Model file for the job. Use its own axes, mm. Face numbers are marked on the shaded views. Round coordinates to 2 decimals unless told otherwise and drop trailing zeros. Write each loop counter-clockwise with the first axis right and the second up, starting at its lowest first coordinate (ties: lowest second). Pieces come first, ordered by that corner, then holes.
Autodesk Fusion 360 part; units mm, degrees
sketch "Sketch1" plane through (0, 0, 0) normal (0, 1, 0) x (1, 0, 0)
  line L0 (0, 0) -> (33.75, 0)
  line L1 (33.75, 0) -> (33.75, -6)
  line L2 (33.75, -6) -> (0, -6)
  line L3 (0, -6) -> (0, 0)
  line L4 (3, -3.9) -> (3, -2.1)
  line L5 (30.75, -2.1) -> (30.75, -3.9)
  line L6 (30.75, -3.9) -> (13.625, -3.9)
  line L7 (12.375, -3.9) -> (3, -3.9)
  line L8 (3, -2.1) -> (12.375, -2.1)
  line L9 (13.625, -2.1) -> (30.75, -2.1)
  arc A0 (12.375, -2.1) -> (13.625, -2.1) centre (13, -2.1) ccw
  arc A1 (12.625, 0) -> (13.375, 0) centre (13, 0) ccw
  arc A2 (13.375, -6) -> (12.625, -6) centre (13, -6) ccw
  arc A3 (13.625, -3.9) -> (12.375, -3.9) centre (13, -3.9) ccw
  dimension "d1" = 33.75
  dimension "d2" = 6
  dimension "d8" = 2.1
  dimension "d9" = 3
  dimension "d10" = 2.1
  dimension "d11" = 3
  dimension "d12" = 27
  dimension "d20" = 10
  dimension "d22" = 10
  dimension "d25" = 0.75
  dimension "d26" = 0.75
  dimension "d27" = 0.625
  dimension "d33" = 1.25
extrude "Extrude1" add sketch "Sketch1" along normal blind 11 contours L0 L1 L2 L3 A1 A2
sketch "Sketch2" plane through (0, 0, 0) normal (0, 0, -1) x (-1, 0, 0)
  line L0 (-33.75, 0) -> (0, 0)
  line L1 (0, 0) -> (0, 11)
  line L2 (0, 11) -> (-33.75, 11)
  line L3 (-33.75, 11) -> (-33.75, 0)
  arc A0 (0, 11) -> (0, 0) centre (12.5393, 5.5) ccw
  line L4 (0, 11) -> (0, 0)
  line L5 (-16.875, 11) -> (-16.875, 0)
  line L6 (-33.75, 11) -> (-33.75, 0)
  arc A1 (-33.75, 0) -> (-33.75, 11) centre (-46.2893, 5.5) ccw
  line L7 (-33.75, 0) -> (-33.75, 11)
extrude "Extrude2" cut sketch "Sketch2" against normal through all contours L3 L6 A1 L7 | L1 A0 L4
fillet "Fillet1" radius 1 2 edges at (0, 11, 3) (0, 0, 3)
fillet "Fillet1" radius 1 2 edges at (33.75, 11, 3) (33.75, 0, 3)
sketch "Sketch3" plane through (0, 11, 0) normal (0, 1, 0) x (-1, 0, 0)
  line L0 (-32.3029, 6) -> (-32.3029, 0)
  line L1 (-32.3029, 0) -> (-1.4471, 0)
  line L2 (-1.4471, 0) -> (-1.4471, 6)
  line L3 (-1.4471, 6) -> (-32.3029, 6)
  line L4 (-30.75, 3.9) -> (-13.625, 3.9)
  line L5 (-3, 3.9) -> (-3, 2.1)
  line L6 (-3, 2.1) -> (-12.375, 2.1)
  arc A0 (-12.375, 2.1) -> (-13.625, 2.1) centre (-13, 2.1) ccw
  line L7 (-13.625, 2.1) -> (-30.75, 2.1)
  line L8 (-30.75, 2.1) -> (-30.75, 3.9)
  circle A1 centre (-13, 0) radius 0.375
  circle A2 centre (-13, 6) radius 0.375
  arc A3 (-13.625, 3.9) -> (-12.375, 3.9) centre (-13, 3.9) ccw
  line L9 (-12.375, 3.9) -> (-3, 3.9)
  dimension "d28" = 0.75
  dimension "d29" = 0.75
  dimension "d30" = 10
  dimension "d31" = 10
extrude "Extrude3" cut sketch "Sketch3" against normal through all contours L3 A2 | L1 A1 picked at (-13.0916, 5.915) picked at (-12.9084, 0.085)
equation "d8 = d10"
equation "d11 = d9"
equation "d25 = d24"
equation "d26 = d24"
equation "d27 = d33 / 2"
equation "d31 = d30"
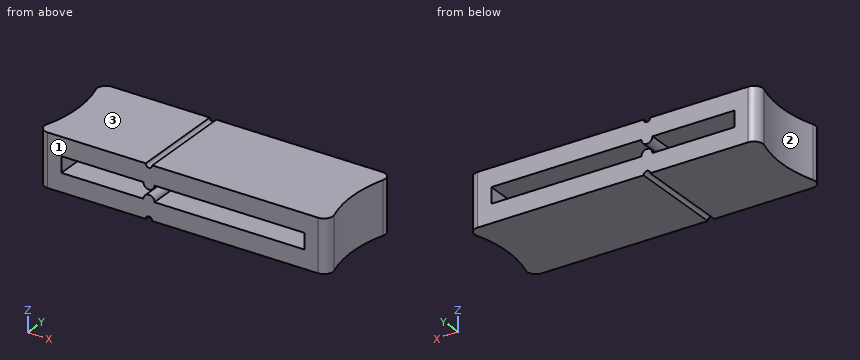
1) Wall check: probe 1 along Z at (x, y) = (15, 1.5); probe 2 along X at (y, z) = (5.25, 3.05); probe 3 along X at (y, z) = (3.5, 3.35). Give the ranges that are in metal, low to high.
2) Cut at B-B on z = 4.55. List the corners of the cut face in (x, y), and give its area (3 significant figures).
3) Pull direction Y, two halves, no side cores. Call the marked faces 1, 2 and 3: released by +Y, released by -Y, zero draft, split by the parting line, or undercut.
4) Cut at D-D on y = 6.75. List the corners of the cut face in (x, z) (3 decimals).
5) Cut at C-C on y = 1. List the corners of the cut face in (x, z) (3 decimals).
6) Flat gauge pins, fed straight in: pin 1 Ø0.9 at (y, z) = (6.5, 3) entering from +X; pin 2 Ø2 at (y, z) = (6, 3) entering from -X. Where does each tip first touch, or does it go through?
7) Cut at A-A on x = 16. List the corners of the cut face in (y, z), and give its area (3 significant figures).
Result sheet:
1. probe 1: z = 0 to 2.1, 3.9 to 6
1. probe 2: x = 1.15 to 3, 30.75 to 32.6
1. probe 3: x = 1.01 to 3, 12.7 to 13.3, 30.75 to 32.74
2. outline: (0.5, 1.31) arc R1 ccw to (1.45, 0) - (32.3, 0) arc R1 ccw to (33.25, 1.31) arc R13.69 cw to (33.25, 9.69) arc R1 ccw to (32.3, 11) - (1.45, 11) arc R1 ccw to (0.5, 9.69) arc R13.69 cw to start
2. area: 352 mm2
3. face 1: released by -Y
3. face 2: undercut
3. face 3: zero draft
4. outline: (1.096, 0) - (12.625, 0) arc R0.375 cw to (13.375, 0) - (32.654, 0) - (32.654, 6) - (13.375, 6) arc R0.375 cw to (12.625, 6) - (1.096, 6) - close; hole (3, 2.1) - (12.375, 2.1) arc R0.625 cw to (13.625, 2.1) - (30.75, 2.1) - (30.75, 3.9) - (13.625, 3.9) arc R0.625 cw to (12.375, 3.9) - (3, 3.9) - close
5. outline: (0.447, 0) - (12.625, 0) arc R0.375 cw to (13.375, 0) - (33.303, 0) - (33.303, 6) - (13.375, 6) arc R0.375 cw to (12.625, 6) - (0.447, 6) - close; hole (3, 2.1) - (12.375, 2.1) arc R0.625 cw to (13.625, 2.1) - (30.75, 2.1) - (30.75, 3.9) - (13.625, 3.9) arc R0.625 cw to (12.375, 3.9) - (3, 3.9) - close
6. pin 1: stops at x = 32.67
6. pin 2: stops at x = 1.07
7. outline: (0, 0) - (11, 0) - (11, 2.1) - (0, 2.1) - close; (0, 3.9) - (11, 3.9) - (11, 6) - (0, 6) - close
7. area: 46.2 mm2
